Design review of the part shown in the three views and the two pictorial views. Dimensions are in mm from the part's minimum x, y and z. A direction names the side the tool comes from. Round coordinates to 2 decimals unless told otherwise and drop trailing zeros. Loops run counter-clockwise (first coordinate to the right, second up) from the corner with the lowest first, then second, coordinate; pieces in that order, holes last. Notation, with made-up numbers: M -23.75,42 L 30.25,42 A10 cw 30.25,51 Z; hole C 7,77 d1. An arc over 180 degrees is marked long. One line per question, with ' | ' between items.
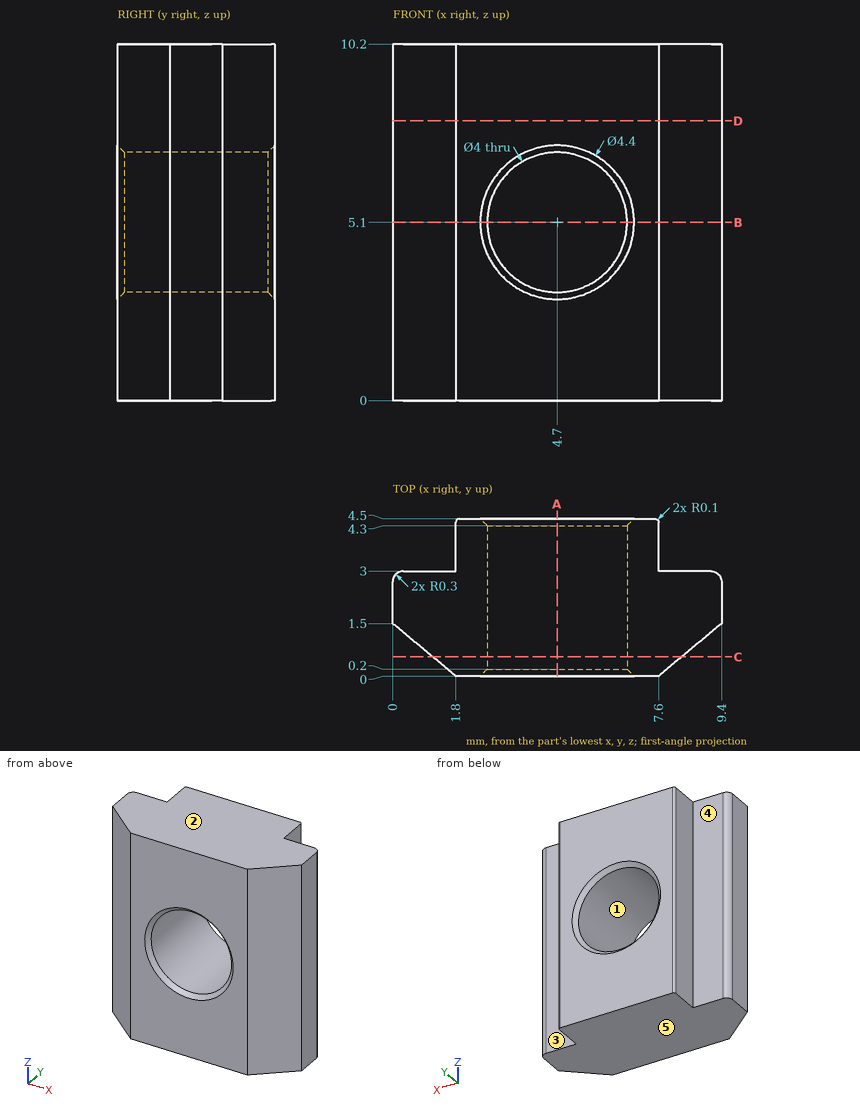
1) Add section A-A on x = 4.7. State the section outline as (y, z) points.
Output values:
outline: M 0,0 L 4.5,0 L 4.5,2.9 L 4.3,3.1 L 0.2,3.1 L 0,2.9 Z; M 0,7.3 L 0.2,7.1 L 4.3,7.1 L 4.5,7.3 L 4.5,10.2 L 0,10.2 Z
2) Add section B-B on z = 5.1. State the section outline as (x, y) points.
Output values:
outline: M 0,1.5 L 1.8,0 L 2.5,0 L 2.7,0.2 L 2.7,4.3 L 2.5,4.5 L 1.9,4.5 A0.1 ccw 1.8,4.4 L 1.8,3 L 0.3,3 A0.3 ccw 0,2.7 Z; M 6.7,0.2 L 6.9,0 L 7.6,0 L 9.4,1.5 L 9.4,2.7 A0.3 ccw 9.1,3 L 7.6,3 L 7.6,4.4 A0.1 ccw 7.5,4.5 L 6.9,4.5 L 6.7,4.3 Z
3) Add section C-C on y = 0.55. State the section outline as (x, z) points, then the cut area to 3 significant figures.
Output values:
outline: M 1.14,0 L 8.26,0 L 8.26,10.2 L 1.14,10.2 Z; hole C 4.7,5.1 d4 | area: 60.1 mm²
4) Mouldability with a two-part tool opening along Z and no side actions: class the marked faces 1, 2 and 3 as +Z half, -Z half, draft (parallel to the pull), parting line (faces both ways), or undercut.
Output values:
face 1: undercut | face 2: +Z half | face 3: draft
5) Machinability: for the marked faces 4 and 5, which of the approach directions +Z, -Z, +X, -X, +Y, -Y give a long, thin tool a straight path to every point of the face, cutting with its end or side? Answer none if there is none.
Output values:
face 4: +Z, -Z, -X, +Y | face 5: -Z, +X, -X, +Y, -Y
6) Add section D-D on z = 8. State the section outline as (x, y) points.
Output values:
outline: M 0,1.5 L 1.8,0 L 7.6,0 L 9.4,1.5 L 9.4,2.7 A0.3 ccw 9.1,3 L 7.6,3 L 7.6,4.4 A0.1 ccw 7.5,4.5 L 1.9,4.5 A0.1 ccw 1.8,4.4 L 1.8,3 L 0.3,3 A0.3 ccw 0,2.7 Z
7) For line 1 (Z direction, x = 4.7, y = 1.2); line 2 (X direction, y = 1.8, z = 5.1); line 3 (X direction, y = 3.35, z = 5.1), list the stretches that pass through material, from the lowest coordinate up.
Output values:
line 1: z = 0 to 3.1, 7.1 to 10.2 | line 2: x = 0 to 2.7, 6.7 to 9.4 | line 3: x = 1.8 to 2.7, 6.7 to 7.6
8) Insertion check: P1, Ø2, axis at x = 5.5, y = 3.5, coming from the -Z side; P2, Ø1.5, axis at y = 4, z = 4, coming from the -X side; P3, Ø0.5, axis at x = 8.5, z = 3.5, coming from the +Y side. Each pin has a flat end and moves straight along its axis. Give the tip position at first contact, or say it passes through.
Output values:
P1: stops at z = 0 | P2: stops at x = 1.8 | P3: stops at y = 3
